Source: CAD feature listing. Evaluate the final solid. Frame: model axes, mm. A direction names the side the tool comes from. Coordinates: 2 decimals unless noted, no trailing zeros. Loops run counter-clockwise (first coordinate to the right, second up) from the corner with the lowest first, then second, coordinate; pieces in that order, holes last.
from build123d import *

# Parameters (mm, degrees)
F0_R     = 25.4
F0_R_2   = 23.749
F1_DEPTH = 254
F2_DEPTH = 254
F4_D     = 19.05
F4_DEPTH = 25.401
F5_D     = 19.05
F5_DEPTH = 25.4010001


with BuildPart() as f1:
    # F0 (on Front) → F1 (new body, symmetric)
    with BuildSketch(Plane.XZ):
        Circle(F0_R)
        Circle(F0_R_2, mode=Mode.SUBTRACT)
    extrude(amount=F1_DEPTH, both=True)

    # F0 (on Front) → F2 (join, symmetric)
    with BuildSketch(Plane.XZ):
        Circle(F0_R)
        Circle(F0_R_2, mode=Mode.SUBTRACT)
    extrude(amount=F2_DEPTH, both=True)

    # F4 (through all, one way)
    with BuildSketch(Plane(origin=(0, 0, 0), x_dir=(1, 0, 0), z_dir=(0, 0, -1))):
        with Locations((0, -203.2)):
            Circle(F4_D / 2)
    extrude(amount=-F4_DEPTH, mode=Mode.SUBTRACT)

    # F5 (through all, one way)
    with BuildSketch(Plane.XY):
        with Locations((0, -203.2)):
            Circle(F5_D / 2)
    extrude(amount=-F5_DEPTH, mode=Mode.SUBTRACT)


solid = f1.part
Q1. Access query for faces 4 (the cylindrical face through (-7.02, 196.76, 23.55)), 5 (the flat face through (17, -254, -17)). Directions: +Z, -Z, +X, -X, +Y, -Y. A direction counts if a zero-diameter tool reaches every point of the face in a straight line with its end or side. Return the directions, or none.
Q2. Section D-D, the plane y = 203.2. Return the cut outline in (x, z) (3 decimals), plus the area to 3 significant figures.
Q3. Section C-C, the plane y = -17. Return the cut outline in (x, z), plus the area to 3 significant figures.
Q4. Draft query along X for faces 1 (the cylindrical face through (-7.02, -196.76, -23.55)), 2 (the cylindrical face through (-5.506, -3.556, -24.796)), 3 (the flat face through (17, 254, -17)). Return one class per face: +X half, -X half, draft (parallel to the pull), parting line (faces both ways), or undercut.
Q5. Section A-A, the plane z = 0. Return the cut outline in (x, y), plus the area to 3 significant figures.
Q6. Section B-B, the plane x = 0. Return the cut outline in (y, z) (3 decimals).
Q7. Line query: line 1 along X through (y, z) = (-98.5, 1); line 2 along Z through (x, y) = (-5, 65); line 3 along X through (y, z) = (32.5, -22). Output: solid intervals per line, ascending.
Q8. Contact query for flat-ended pins moving along their axis: pin 1 Ø25 at (x, y) = (0, 203.2) entering from -Z; pin 2 Ø5 at (y, z) = (132.5, 11) entering from -X; pin 3 Ø6 at (x, y) = (-7.5, 141) entering from +Z. Output: stop coordinate, or through.
Derived:
1. face 4: +Z
1. face 5: +Z, -Z, +X, -X, -Y
2. outline: (-9.525, 21.755) - (-9.525, 23.546) arc R25.4 ccw (long way) to (9.525, 23.546) - (9.525, 21.755) arc R23.749 cw (long way) to start
2. area: 223 mm2
3. outline: circle Ø50.8 at (0, 0); hole circle Ø47.5 at (0, 0)
3. area: 255 mm2
4. face 1: undercut
4. face 2: parting line
4. face 3: draft
5. outline: (-25.4, -254) - (-23.75, -254) - (-23.75, 254) - (-25.4, 254) - close; (23.75, -254) - (25.4, -254) - (25.4, 254) - (23.75, 254) - close
5. area: 1,680 mm2
6. outline: (-254, -25.4) - (-212.725, -25.4) - (-212.725, -23.749) - (-254, -23.749) - close; (-254, 23.749) - (193.675, 23.749) - (193.675, 25.4) - (-254, 25.4) - close; (-193.675, -25.4) - (254, -25.4) - (254, -23.749) - (-193.675, -23.749) - close; (212.725, 23.749) - (254, 23.749) - (254, 25.4) - (212.725, 25.4) - close
7. line 1: x = -25.38 to -23.73, 23.73 to 25.38
7. line 2: z = -24.9 to -23.22, 23.22 to 24.9
7. line 3: x = -12.69 to -8.95, 8.95 to 12.69
8. pin 1: stops at z = -25.4
8. pin 2: stops at x = -23.94
8. pin 3: stops at z = 25
